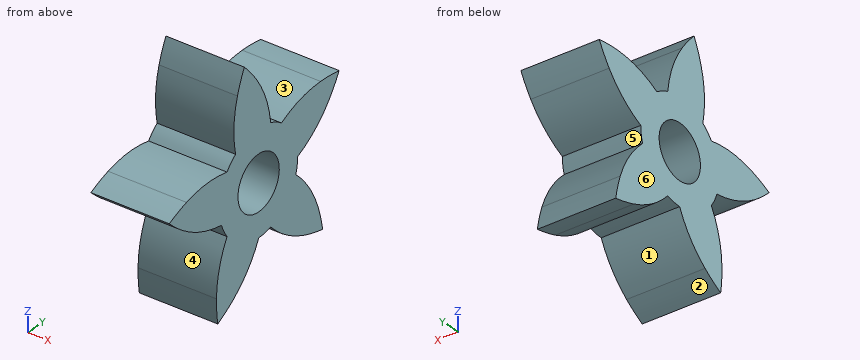
```python
from build123d import *

# Parameters (mm, degrees)
SKETCH1_R                = 2.75
BOSS_EXTRUDE1_DEPTH      = 4
BOSS_EXTRUDE1_DEPTH_BACK = 4


with BuildPart() as part:
    # Sketch1 → Boss-Extrude1 (new body, two sides)
    with BuildSketch(Plane(origin=(0, 0, 0), x_dir=(0, 0, -1), z_dir=(1, 0, 0))) as boss_extrude1_sk:
        with BuildLine():
            ThreePointArc((6.104566947, 7.920496348), (3.660962149, 6.718169615), (1.588390796, 4.951465912))
            ThreePointArc((1.588390796, 4.951465912), (0.803858587, 5.137490766), (0, 5.2))
            ThreePointArc((0, 5.2), (-1.433855865, 7.515351235), (-3.393406085, 9.406635697))
            ThreePointArc((-3.393406085, 9.406635697), (-4.411888917, 10.105404063), (-5.485434516, 10.716210377))
            ThreePointArc((-5.485434516, 10.716210377), (-5.617706577, 9.488167784), (-5.646424734, 8.253356149))
            ThreePointArc((-5.646424734, 8.253356149), (-5.25805947, 5.557810489), (-4.218284171, 3.040736531))
            ThreePointArc((-4.218284171, 3.040736531), (-4.637638106, 2.352086903), (-4.945493885, 1.606888371))
            ThreePointArc((-4.945493885, 1.606888371), (-7.590609594, 0.958693286), (-9.994862325, -0.32051068))
            ThreePointArc((-9.994862325, -0.32051068), (-10.974159037, -1.073214113), (-11.886814196, -1.90546712))
            ThreePointArc((-11.886814196, -1.90546712), (-10.759750601, -2.410751356), (-9.594249347, -2.819641726))
            ThreePointArc((-9.594249347, -2.819641726), (-6.910621616, -3.283253829), (-4.195433788, -3.072187385))
            ThreePointArc((-4.195433788, -3.072187385), (-3.670076564, -3.683821116), (-3.056483312, -4.206888371))
            ThreePointArc((-3.056483312, -4.206888371), (-3.257398859, -6.922846199), (-2.783758545, -9.604722191))
            ThreePointArc((-2.783758545, -9.604722191), (-2.370514366, -10.768686862), (-1.861020675, -11.893853821))
            ThreePointArc((-1.861020675, -11.893853821), (-1.032185004, -10.978094061), (-0.283147459, -9.995990572))
            ThreePointArc((-0.283147459, -9.995990572), (0.987060428, -7.586972949), (1.625363492, -4.939452755))
            ThreePointArc((1.625363492, -4.939452755), (2.369406048, -4.628813561), (3.056483312, -4.206888371))
            ThreePointArc((3.056483312, -4.206888371), (5.577426384, -5.237247536), (8.274404928, -5.615534087))
            ThreePointArc((8.274404928, -5.615534087), (9.509100588, -5.582200382), (10.736640165, -5.445338799))
            ThreePointArc((10.736640165, -5.445338799), (10.121825185, -4.374083905), (9.419254594, -3.358220198))
            ThreePointArc((9.419254594, -3.358220198), (7.520658509, -1.405753325), (5.199963671, 0.019437697))
            ThreePointArc((5.199963671, 0.019437697), (5.134450035, 0.823057007), (4.945493885, 1.606888371))
            ThreePointArc((4.945493885, 1.606888371), (6.704437934, 3.686049214), (7.897622027, 6.13413126))
            ThreePointArc((7.897622027, 6.13413126), (8.247461732, 7.318697294), (8.496629222, 8.528449363))
            ThreePointArc((8.496629222, 8.528449363), (7.287816997, 8.274761538), (6.104566947, 7.920496348))
        make_face()
        Circle(SKETCH1_R, mode=Mode.SUBTRACT)
    extrude(amount=BOSS_EXTRUDE1_DEPTH)
    extrude(boss_extrude1_sk.sketch, amount=-BOSS_EXTRUDE1_DEPTH_BACK)


solid = part.part
```
Geometry: final body of the model. Coordinates: model frame, mm. Face numbers are marked on the shaded views. A direction names the side the tool comes from. Coordinates: 2 decimals unless noted, no trailing zeros. Order: outer loops, then holes, each group sorted by start corner. A loop starts at its lowest first (then second) coordinate and runs counter-clockwise, first axis right, second up. Notation, with made-up numbers: (12.5, 76.25) -> (60.5, 76.25) arc R25 ccw to (60.5, 107.25) -> close; hole circle Ø6 at (-7.5, 44). An arc over 180 degrees is marked (long way). Use CSV: the item, a comma, the result in double quotes.
1) Section C-C on z = -7.5. Output: boundary loops of the cut face in (x, y).
Findings:
outline,"(-4, -5.58) -> (4, -5.58) -> (4, -1.39) -> (-4, -1.39) -> close; (-4, 5.13) -> (4, 5.13) -> (4, 8.33) -> (-4, 8.33) -> close"
2) Access query for the marked faces 5 and 6. Directions: +Z, -Z, +X, -X, +Y, -Y. A direction counts if a zero-diameter tool reaches every point of the face in a straight line with its end or side. Return the directions, or none.
Findings:
face 5,"+X, -X, +Y"
face 6,"+Z, -Z, -X, +Y, -Y"
3) Mould query, pull axis Y, two halves, no side actions, for the marked faces 1, 2, 3 and 4. Classes: +Y half, -Y half, draft (parallel to the pull), parting line (faces both ways), or undercut.
Findings:
face 1,"undercut"
face 2,"+Y half"
face 3,"undercut"
face 4,"-Y half"
4) Section D-D on y = -8. Output: boundary loops of the cut face in (x, z), then the cut area to 3 significant figures.
Findings:
outline,"(-4, -0.82) -> (4, -0.82) -> (4, 3.15) -> (-4, 3.15) -> close"
area,"31.8 mm^2"
5) Section A-A on x = 3.5. Output: boundary loops of the cut face in (y, z).
Findings:
outline,"(-11.89, 1.86) arc R14.7 ccw to (-10, 0.28) arc R10.98 ccw to (-4.94, -1.63) arc R5.2 ccw to (-4.21, -3.06) arc R10.98 ccw to (-5.62, -8.27) arc R14.7 ccw to (-5.45, -10.74) arc R14.7 ccw to (-3.36, -9.42) arc R10.98 ccw to (0.02, -5.2) arc R5.2 ccw to (1.61, -4.95) arc R10.98 ccw to (6.13, -7.9) arc R14.7 ccw to (8.53, -8.5) arc R14.7 ccw to (7.92, -6.1) arc R10.98 ccw to (4.95, -1.59) arc R5.2 ccw to (5.2, 0) arc R10.98 ccw to (9.41, 3.39) arc R14.7 ccw to (10.72, 5.49) arc R14.7 ccw to (8.25, 5.65) arc R10.98 ccw to (3.04, 4.22) arc R5.2 ccw to (1.61, 4.95) arc R10.98 ccw to (-0.32, 9.99) arc R14.7 ccw to (-1.91, 11.89) arc R14.7 ccw to (-2.82, 9.59) arc R10.98 ccw to (-3.07, 4.2) arc R5.2 ccw to (-4.21, 3.06) arc R10.98 ccw to (-9.6, 2.78) arc R14.7 ccw to start; hole circle Ø5.5 at (0, 0)"
6) Pin query (flat end, axial travel): pin 1 Ø4 at (x, z) = (-1, 1.5) entering from +Y. Return the tip coordinate at first contact, or that it passes through.
Findings:
pin 1,"stops at y = 9.49"
7) Section B-B on y = 2. Output: boundary loops of the cut face in (x, z).
Findings:
outline,"(-4, -5.35) -> (4, -5.35) -> (4, -1.89) -> (-4, -1.89) -> close; (-4, 1.89) -> (4, 1.89) -> (4, 4.8) -> (-4, 4.8) -> close"
8) Line query: line 1 (Z direction, x = 1.25, y = -1.5); line 2 (Z direction, x = 1.5, y = -1); line 3 (Z direction, x = -2, y = 4.25). Output: solid intervals per line, ascending.
Findings:
line 1,"z = -7.64 to -2.3, 2.3 to 11.46"
line 2,"z = -6.98 to -2.56, 2.56 to 10.89"
line 3,"z = -7.05 to 4.81"
